Here's how the part is built. I have some questions about the finished solid (model axes, mm). A direction names the side the tool comes from. Coordinates: 2 decimals unless noted, no trailing zeros. Write each loop counter-clockwise with the first axis right and the second up, starting at its lowest first coordinate (ties: lowest second). Pieces come first, ordered by that corner, then holes.
from build123d import *

# Parameters (mm, degrees)
SKETCH1_R           = 32.5
BOSS_EXTRUDE1_DEPTH = 80
SKETCH2_R           = 32.5
BOSS_EXTRUDE2_DEPTH = 12.5
SKETCH6_R           = 32.5
BOSS_EXTRUDE4_DEPTH = 12.5


with BuildPart() as part:
    # Sketch1 → Boss-Extrude1 (new body)
    with BuildSketch(Plane.XY):
        with BuildLine():
            Line((-225.792643224, 137.875019839), (-173.792643224, 137.875019839))
            ThreePointArc((-173.792643224, 137.875019839), (-133.792643224, 97.875019839), (-173.792643224, 57.875019839))
            Line((-173.792643224, 57.875019839), (-225.792643224, 57.875019839))
            Line((-225.792643224, 57.875019839), (-225.792643224, 137.875019839))
        make_face()
        with Locations((-177.792643224, 97.875019839)):
            Circle(SKETCH1_R, mode=Mode.SUBTRACT)
    extrude(amount=BOSS_EXTRUDE1_DEPTH)

    # Sketch2 → Boss-Extrude2 (add)
    with BuildSketch(Plane.XY.offset(80)):
        with BuildLine():
            Line((-173.792643224, 49.875019839), (-233.792643224, 49.875019839))
            Line((-233.792643224, 49.875019839), (-233.792643224, 145.875019839))
            Line((-233.792643224, 145.875019839), (-173.792643224, 145.875019839))
            ThreePointArc((-173.792643224, 145.875019839), (-125.792643224, 97.875019839), (-173.792643224, 49.875019839))
        make_face()
        with BuildLine():
            Line((-225.792643224, 137.875019839), (-225.792643224, 57.875019839))
            Line((-225.792643224, 57.875019839), (-173.792643224, 57.875019839))
            ThreePointArc((-173.792643224, 57.875019839), (-133.792643224, 97.875019839), (-173.792643224, 137.875019839))
            Line((-173.792643224, 137.875019839), (-225.792643224, 137.875019839))
        make_face(mode=Mode.SUBTRACT)
        with BuildLine():
            Line((-173.792643224, 137.875019839), (-225.792643224, 137.875019839))
            Line((-225.792643224, 137.875019839), (-225.792643224, 57.875019839))
            Line((-225.792643224, 57.875019839), (-173.792643224, 57.875019839))
            ThreePointArc((-173.792643224, 57.875019839), (-133.792643224, 97.875019839), (-173.792643224, 137.875019839))
        make_face()
        with Locations((-177.792643224, 97.875019839)):
            Circle(SKETCH2_R, mode=Mode.SUBTRACT)
    extrude(amount=BOSS_EXTRUDE2_DEPTH)

    # Sketch6 → Boss-Extrude4 (add)
    with BuildSketch(Plane(origin=(0, 0, 0), x_dir=(-1, 0, 0), z_dir=(0, 0, -1))):
        with BuildLine():
            Line((233.792643224, 145.875019839), (173.792643224, 145.875019839))
            ThreePointArc((173.792643224, 145.875019839), (125.792643224, 97.875019839), (173.792643224, 49.875019839))
            Line((173.792643224, 49.875019839), (233.792643224, 49.875019839))
            Line((233.792643224, 49.875019839), (233.792643224, 145.875019839))
        make_face()
        with Locations((177.792643224, 97.875019839)):
            Circle(SKETCH6_R, mode=Mode.SUBTRACT)
    extrude(amount=BOSS_EXTRUDE4_DEPTH)


solid = part.part
1. If I drill on line 1 (Z direction, x = -150.5, y = 133); line 2 (X direction, y = 97, z = 61); line 3 (X direction, y = 80.5, z = -5), over which ranges is the centre line in solid material (lowest first)?
2. On a 3-axis mill with a long thin cutter (end or side, diameter ignored), from which of +Z, -Z, +X, -X, +Y, -Y can I reach the whole of each face in a straight line? I mean faces 4 (the face through (-199, 57.875, 39)), 5 (the face through (-225.793, 97, 39)), 6 (the face through (-125.804, 98.931, -6.162)), 7 (the face through (-133.802, 98.755, 39.44)), 8 (the face through (-184, 141, 0)). Say none if no direction works.
3. I want a section at C-C (x = -223). List the corners of the cut face in (y, z) for me.
4. I want a section at D-D (z = 37.5). List the corners of the cut face in (x, y) for me, then the cut area to 3 significant figures.
5. For pin 1 Ø6 at (x, z) = (-212.5, 31) entering from +Y (3 decimals); pin 2 Ø1 at (y, z) = (103, 43) entering from -X; pin 3 Ø1 at (y, z) = (75.5, 3.5) entering from +X, each with a flat end and sliding along its axis, tell me the tip position at first contact or that it passes through.
6. Thinking about a two-plate mould opening in Z: for faces 1 (the face through (-125.804, 98.931, 86.162)), 2 (the face through (-200, 137.875, 39)), 3 (the face through (-203, 120, 92.5)), which applies, pulls with the +Z half, pulls with the -Z half, needs draft (parallel to the pull), parting line crosses it, or undercut?
7. I want a section at B-B (x = -179.5). List the corners of the cut face in (y, z) for me.
8. I want a section at A-A (y = 116). List the corners of the cut face in (x, z) for me.
Response values:
1. line 1: z = -12.5 to 0, 80 to 92.5
1. line 2: x = -225.79 to -210.28, -145.3 to -133.8
1. line 3: x = -233.79 to -205.26, -150.33 to -129.05
2. face 4: +X, -X, -Y
2. face 5: -X, +Y, -Y
2. face 6: +Z, -Z, +X
2. face 7: +X
2. face 8: none
3. outline: (49.88, -12.5) - (145.88, -12.5) - (145.88, 0) - (137.88, 0) - (137.88, 80) - (145.88, 80) - (145.88, 92.5) - (49.88, 92.5) - (49.88, 80) - (57.88, 80) - (57.88, 0) - (49.88, 0) - close
4. outline: (-225.79, 57.88) - (-173.79, 57.88) arc R40 ccw to (-173.79, 137.88) - (-225.79, 137.88) - close; hole circle Ø65 at (-177.79, 97.88)
4. area: 3,350 mm2
5. pin 1: stops at y = 137.875
5. pin 2: stops at x = -225.79
5. pin 3: stops at x = -140.3
6. face 1: needs draft
6. face 2: undercut
6. face 3: pulls with the +Z half
7. outline: (49.88, -12.5) - (65.42, -12.5) - (65.42, 92.5) - (49.88, 92.5) - (49.88, 80) - (57.88, 80) - (57.88, 0) - (49.88, 0) - close; (130.33, -12.5) - (145.88, -12.5) - (145.88, 0) - (137.88, 0) - (137.88, 80) - (145.88, 80) - (145.88, 92.5) - (130.33, 92.5) - close
8. outline: (-233.79, -12.5) - (-204.77, -12.5) - (-204.77, 92.5) - (-233.79, 92.5) - (-233.79, 80) - (-225.79, 80) - (-225.79, 0) - (-233.79, 0) - close; (-150.82, -12.5) - (-129.35, -12.5) - (-129.35, 0) - (-138.13, 0) - (-138.13, 80) - (-129.35, 80) - (-129.35, 92.5) - (-150.82, 92.5) - close
